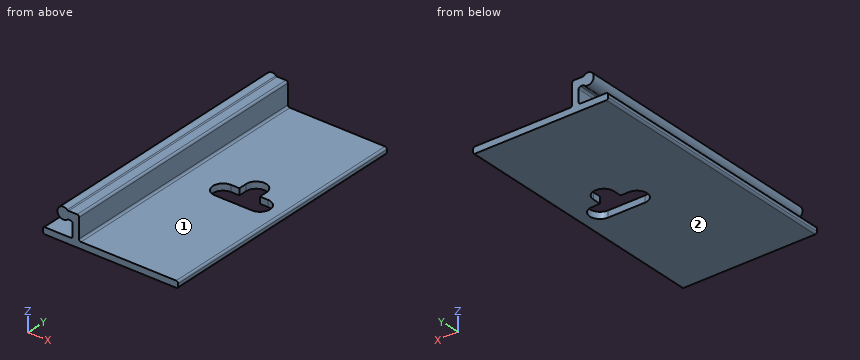
```python
from build123d import *

# Parameters (mm, degrees)
BOSS_EXTRUDE1_DEPTH = 50.8
SKETCH4_W           = 2.921
SKETCH4_H           = 4.572
CUT_EXTRUDE2_DEPTH  = 51.8
FILLET1_R           = 0.381
CUT_EXTRUDE1_DEPTH  = 2.27


with BuildPart() as part:
    # Sketch2 → Boss-Extrude1 (new body)
    with BuildSketch(Plane(origin=(0, 0, 0), x_dir=(1, 0, 0), z_dir=(0, 1, 0))):
        with BuildLine():
            Line((-5.969, 0), (19.431, 0))
            ThreePointArc((19.431, 0), (19.700407684, -0.111592316), (19.812, -0.381))
            Line((19.812, -0.381), (19.812, -0.889))
            ThreePointArc((19.812, -0.889), (19.700407684, -1.158407684), (19.431, -1.27))
            Line((19.431, -1.27), (1.016, -1.27))
            ThreePointArc((1.016, -1.27), (0.746592316, -1.381592316), (0.635, -1.651))
            Line((0.635, -1.651), (0.635, -3.937))
            ThreePointArc((0.635, -3.937), (0.746592316, -4.206407684), (1.016, -4.318))
            Line((1.016, -4.318), (1.40496875, -4.318))
            ThreePointArc((1.40496875, -4.318), (1.539672592, -4.293392866), (1.656976563, -4.22275))
            ThreePointArc((1.656976563, -4.22275), (3.556, -5.08), (1.656976563, -5.93725))
            ThreePointArc((1.656976563, -5.93725), (1.539672592, -5.866607134), (1.40496875, -5.842))
            Line((1.40496875, -5.842), (-1.40496875, -5.842))
            ThreePointArc((-1.40496875, -5.842), (-1.539672592, -5.866607134), (-1.656976563, -5.93725))
            ThreePointArc((-1.656976563, -5.93725), (-3.556, -5.08), (-1.656976563, -4.22275))
            ThreePointArc((-1.656976563, -4.22275), (-1.539672592, -4.293392866), (-1.40496875, -4.318))
            Line((-1.40496875, -4.318), (-1.016, -4.318))
            ThreePointArc((-1.016, -4.318), (-0.746592316, -4.206407684), (-0.635, -3.937))
            Line((-0.635, -3.937), (-0.635, -1.651))
            ThreePointArc((-0.635, -1.651), (-0.746592316, -1.381592316), (-1.016, -1.27))
            Line((-1.016, -1.27), (-5.969, -1.27))
            ThreePointArc((-5.969, -1.27), (-6.238407684, -1.158407684), (-6.35, -0.889))
            Line((-6.35, -0.889), (-6.35, -0.381))
            ThreePointArc((-6.35, -0.381), (-6.238407684, -0.111592316), (-5.969, 0))
        make_face()
    extrude(amount=BOSS_EXTRUDE1_DEPTH)

    # Sketch4 → Cut-Extrude2 (cut, through all)
    with BuildSketch(Plane.XZ):
        with Locations((2.0955, 3.937)):
            Rectangle(SKETCH4_W, SKETCH4_H)
    extrude(amount=-CUT_EXTRUDE2_DEPTH, mode=Mode.SUBTRACT)

    # Fillet1
    fillet1_edges = [part.edges().sort_by_distance(p)[0] for p in [
        (0.635, 25.4, 5.842),
    ]]
    fillet(fillet1_edges, radius=FILLET1_R)

    # Sketch3 → Cut-Extrude1 (cut, through all)
    with BuildSketch(Plane.XY.offset(1.27)):
        with BuildLine():
            Line((8.2931, 27.3812), (9.8806, 27.3812))
            Line((9.8806, 27.3812), (9.8806, 28.9814))
            ThreePointArc((9.8806, 28.9814), (11.8618, 30.9626), (13.843, 28.9814))
            Line((13.843, 28.9814), (13.843, 27.3812))
            Line((13.843, 27.3812), (15.4305, 27.3812))
            ThreePointArc((15.4305, 27.3812), (17.4117, 25.4), (15.4305, 23.4188))
            Line((15.4305, 23.4188), (8.2931, 23.4188))
            ThreePointArc((8.2931, 23.4188), (6.3119, 25.4), (8.2931, 27.3812))
        make_face()
    extrude(amount=-CUT_EXTRUDE1_DEPTH, mode=Mode.SUBTRACT)


solid = part.part
```
Here's how the part is built. I have some questions about the finished solid (model axes, mm). Face numbers are marked on the shaded views. A direction names the side the tool comes from. Round coordinates to 2 decimals unless told otherwise and drop trailing zeros. Order: outer loops, then holes, each group sorted by start corner. A loop starts at its lowest first (then second) coordinate and runs counter-clockwise, first axis right, second up. Notation, with made-up numbers: (9.25, -5) -> (27.25, -5) arc R23 ccw to (27.25, 9) -> close; hole circle Ø4 at (12.5, 43.25). An arc over 180 degrees is marked (long way). Use a Markdown table: item, result. Add a question column.
(1) For the marked faces 1 and 2, which set-ups out of +Z, -Z, +X, -X, +Y, -Y let a thin tool reach every point of the face, with its end or its side?
(2) I need wall thicknesses on line 1 along Z through (x, y) = (-2.5, 20.5); line 2 along Z through (x, y) = (-5, 14); line 3 along X through (y, z) = (24, 3) (3 decimals). Which ranges of each line are inside material? Lowest first, please.
(3) For pin 1 Ø1.1 at (y, z) = (16, 3) entering from -X (3 decimals); pin 2 Ø1.9 at (y, z) = (18, 3.5) entering from +X (3 decimals); pin 3 Ø1.8 at (x, y) = (-1, 18.5) entering from +Z; pin 4 Ø1 at (y, z) = (28.5, 1) entering from +X, each with a flat end and sliding along its axis, tell me the tip position at first contact or that it passes through.
(4) Suppose I cut it at B-B, the plane x = 16. Please give me the cut outline in (y, z).
(5) Suppose I cut it at C-C, the plane y = 5. Please give me the cut outline in (x, z) (3 decimals), and give its area (3 significant figures).
(6) Suppose I cut it at A-A, the plane y = 25.4. Please give me the cut outline in (x, z) (3 decimals).
Verdict:
| question | item | result |
|---|---|---|
| 1 | face 1 | +Z, +X, +Y, -Y |
| 1 | face 2 | -Z, +X, -X, +Y, -Y |
| 2 | line 1 | 0 to 1.27, 3.94 to 6.22 |
| 2 | line 2 | 0 to 1.27 |
| 2 | line 3 | -0.635 to 0.635 |
| 3 | pin 1 | x = -0.635 |
| 3 | pin 2 | x = 0.635 |
| 3 | pin 3 | z = 6.1 |
| 3 | pin 4 | x = 19.81 |
| 4 | outline | (0, 0) -> (23.5, 0) -> (23.5, 1.27) -> (0, 1.27) -> close; (27.3, 0) -> (50.8, 0) -> (50.8, 1.27) -> (27.3, 1.27) -> close |
| 5 | outline | (-6.35, 0.381) arc R0.381 ccw to (-5.969, 0) -> (19.431, 0) arc R0.381 ccw to (19.812, 0.381) -> (19.812, 0.889) arc R0.381 ccw to (19.431, 1.27) -> (1.016, 1.27) arc R0.381 cw to (0.635, 1.651) -> (0.635, 5.461) arc R0.381 ccw to (0.254, 5.842) -> (-1.405, 5.842) arc R0.381 cw to (-1.657, 5.937) arc R1.143 ccw (long way) to (-1.657, 4.223) arc R0.381 cw to (-1.405, 4.318) -> (-1.016, 4.318) arc R0.381 cw to (-0.635, 3.937) -> (-0.635, 1.651) arc R0.381 cw to (-1.016, 1.27) -> (-5.969, 1.27) arc R0.381 ccw to (-6.35, 0.889) -> close |
| 5 | area | 44.2 mm2 |
| 6 | outline | (-6.35, 0.381) arc R0.381 ccw to (-5.969, 0) -> (6.312, 0) -> (6.312, 1.27) -> (1.016, 1.27) arc R0.381 cw to (0.635, 1.651) -> (0.635, 5.461) arc R0.381 ccw to (0.254, 5.842) -> (-1.405, 5.842) arc R0.381 cw to (-1.657, 5.937) arc R1.143 ccw (long way) to (-1.657, 4.223) arc R0.381 cw to (-1.405, 4.318) -> (-1.016, 4.318) arc R0.381 cw to (-0.635, 3.937) -> (-0.635, 1.651) arc R0.381 cw to (-1.016, 1.27) -> (-5.969, 1.27) arc R0.381 ccw to (-6.35, 0.889) -> close; (17.412, 0) -> (19.431, 0) arc R0.381 ccw to (19.812, 0.381) -> (19.812, 0.889) arc R0.381 ccw to (19.431, 1.27) -> (17.412, 1.27) -> close |
